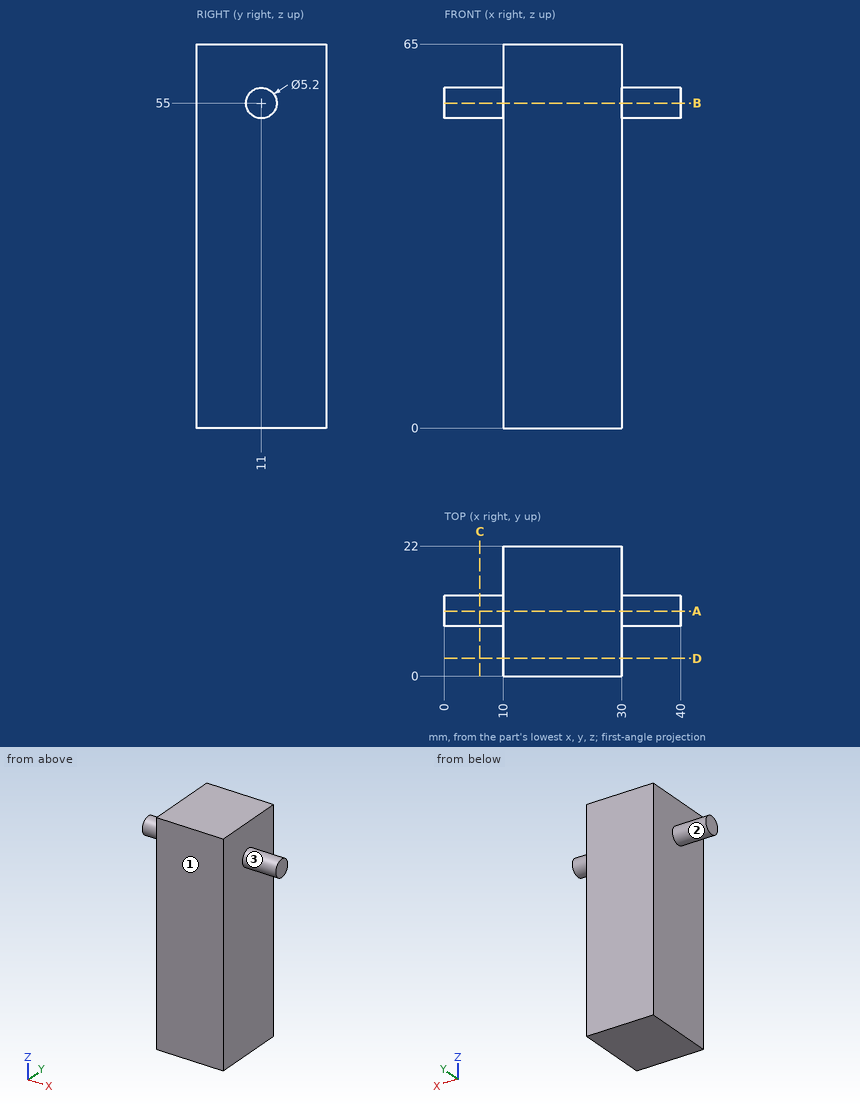
Input: dimensioned drawing with shaded views. Units: mm. Origin: part minimum x, y, z. A direction names the side the tool comes from. Give positions to 0.01 mm unless a question says otherwise; leave off trailing zeros. Loops run counter-clockwise (first coordinate to the right, second up) from the corner with the lowest first, then second, coordinate; pieces in that order, holes last. Notation, with made-up numbers: M 36.5,66 L 55.5,66 A27 cw 55.5,88 Z; hole C 2,36.5 d2. An arc over 180 degrees is marked long. Put each result on its own line as item: value.
1) Cut plane C-C, the plane x = 6. Return the cut outline in (y, z).
Computed values:
outline: C 11,55 d5.2
2) Cut plane A-A, the plane y = 11. Return the cut outline in (x, z).
Computed values:
outline: M 0,52.4 L 10,52.4 L 10,0 L 30,0 L 30,52.4 L 40,52.4 L 40,57.6 L 30,57.6 L 30,65 L 10,65 L 10,57.6 L 0,57.6 Z
3) Material intervals for L1, parallel to X at y = 9, z = 47.5; L2, parallel to Z at x = 38.5, y = 12; L3, parallel to Z at x = 3, y = 13.25, sorted ascending. Write a range as from..to.
Computed values:
L1: x = 10..30
L2: z = 52.6..57.4
L3: z = 53.7..56.3
4) Reachability of the marked faces 1, 2 and 3 from +Z, -Z, +X, -X, +Y, -Y: full face, straight path, thin tool, end or side. Return the list, or none.
Computed values:
face 1: +Z, -Z, +X, -X, -Y
face 2: -X
face 3: +X
5) Cut plane B-B, the plane z = 55. Return the cut outline in (x, y), plus the area to 3 significant figures.
Computed values:
outline: M 0,8.4 L 10,8.4 L 10,0 L 30,0 L 30,8.4 L 40,8.4 L 40,13.6 L 30,13.6 L 30,22 L 10,22 L 10,13.6 L 0,13.6 Z
area: 544 mm^2
6) Cut plane D-D, the plane y = 3. Return the cut outline in (x, z), plus the area to 3 significant figures.
Computed values:
outline: M 10,0 L 30,0 L 30,65 L 10,65 Z
area: 1,300 mm^2
7) First-contact query: P1, Ø6, axis at y = 15, z = 16, coming from the -X side; P2, Ø12, axis at y = 10, z = 22, coming from the +X side; P3, Ø1.5, axis at x = 14, y = 3, coming from the -Z side. Flat tips, straight axial feed; report the tip coordinate or a pass-through.
Computed values:
P1: stops at x = 10
P2: stops at x = 30
P3: stops at z = 0
